Autodesk Inventor part; units mm, degrees
ref_plane "YZ Plane" through (0, 0, 0) normal (1, 0, 0) x (0, 1, 0)
ref_plane "XZ Plane" through (0, 0, 0) normal (0, 1, 0) x (-1, 0, 0)
ref_plane "XY Plane" through (0, 0, 0) normal (0, 0, 1) x (1, 0, 0)
sketch "Sketch3" plane through (0, 0, 0) normal (0, 0, 1) x (1, 0, 0)
  circle A0 centre (1.4019, 6.1779) radius 2.1844
  circle A1 centre (-11.2981, 6.1779) radius 2.1844
  circle A2 centre (-23.9981, 6.1779) radius 2.1844
  circle A3 centre (14.1019, 6.1779) radius 2.1844
  line L0 (-11.2981, 6.1779) -> (1.4019, 6.1779)
  line L1 (1.4019, 6.1779) -> (14.1019, 6.1779)
  circle A4 centre (-11.2981, 6.1779) radius 5.08
  circle A5 centre (1.4019, 6.1779) radius 5.08
  circle A6 centre (14.1019, 6.1779) radius 5.08
  line L2 (-11.2981, 11.2579) -> (1.4019, 11.2579)
  line L3 (1.4019, 11.2579) -> (14.1019, 11.2579)
  line L4 (1.4019, 6.1779) -> (1.4019, -6.5221)
  circle A7 centre (1.4019, -6.5221) radius 2.54
  circle A8 centre (1.4019, -6.5221) radius 5.08
  line L5 (-2.0302, -10.2675) -> (-18.1161, 5.8501)
  line L6 (5.1405, -9.9615) -> (17.9077, 2.813)
  point P0 (0, 0)
  point P1 (-15.8845, 3.9935)
  point P2 (18.6882, 3.9935)
  point P3 (4.8339, -10.2675)
  point P4 (-14.5389, 2.2658)
  point P5 (17.3918, 2.2658)
  point P6 (1.4019, -1.4421)
  point P7 (1.4019, 1.0979)
  point P8 (6.4819, 6.1779)
  point P9 (9.0219, 6.1779)
  point P10 (17.4689, 2.374)
  point P11 (-2.3502, -9.9468)
  point P12 (-15.2165, 2.9448)
  point P13 (-3.6781, 6.1779)
  point P14 (-6.2181, 6.1779)
  dimension "d55" = 10.16
  dimension "d54" = 10.16
  dimension "d56" = 10.16
  dimension "d59" = 4.3688
  dimension "d63" = 12.7
  dimension "d64" = 5.08
  dimension "d65" = 10.16
extrude "Extrusion7" add sketch "Sketch3" along normal blind 1.5875 contours L1 A5 L4 A0 | A0 L0 A5 L1 | A0 L4 A5 L0 | A5 L3 A6 L1 | L1 A6 L6 A8 L4 A5 | A8 | A5 L4 A8 L5 A4 L0 | L0 A4 L2 A5 | A6 L6 | A4 L5 picked at (18.1676, 5.7732) picked at (-7.2265, 5.798)
sketch "Sketch4" plane through (0, 0, 1.5875) normal (0, 0, 1) x (1, 0, 0)
  point P0 (0, 0)
properties part number "Wing poly connection"
The model under review builds one solid part; all positions refer to its coordinate system, in mm. Round coordinates to 2 decimals unless told otherwise and drop trailing zeros. Loops run counter-clockwise (first coordinate to the right, second up) from the corner with the lowest first, then second, coordinate; pieces in that order, holes last. Notation, with made-up numbers: (19, 2.25) -> (23, 2.25) arc R19 cw to (23, 32.25) -> close; hole circle Ø11 at (-1, 34.5). An arc over 180 degrees is marked (long way). One line per question, with ' | ' between items. Start each with the question number.
Item 1: Add section C-C, the plane x = 13. Write out the cut boundary in (y, z), then the cut area to 3 significant figures.
Item 2: Add section A-A, the plane y = -7. Write out the cut boundary in (x, z), then the cut area to 3 significant figures.
Item 3: For pin 1 (4 mm diameter, centred on x = 2, y = -8, fed in from -Z), flat-tipped, find the tip position at first contact; note if it passes through.
Item 4: Add section D-D, the plane z = 1.2. Write out the cut boundary in (x, y).
Item 5: Add section B-B, the plane y = 5.5. Write out the cut boundary in (x, z).
Item 6: Wall thickness on line 1 along Y through (x, z) = (2.5, 0.4); line 2 along X through (y, z) = (7.25, 1.4); line 3 along Y through (x, z) = (3, 0.75): over which ranges is each line inside the solid? List them lowest first. Write a range as [from, to].
Return value:
1) outline: (-2.1, 0) -> (4.29, 0) -> (4.29, 1.59) -> (-2.1, 1.59) -> close; (8.06, 0) -> (11.26, 0) -> (11.26, 1.59) -> (8.06, 1.59) -> close | area: 15.2 mm2
2) outline: (-5.29, 0) -> (-1.09, 0) -> (-1.09, 1.59) -> (-5.29, 1.59) -> close; (3.9, 0) -> (8.1, 0) -> (8.1, 1.59) -> (3.9, 1.59) -> close | area: 13.3 mm2
3) pin 1: stops at z = 0
4) outline: (-15.22, 2.94) -> (-2.03, -10.27) arc R5.08 ccw to (5.14, -9.96) -> (17.91, 2.81) arc R5.08 ccw to (14.1, 11.26) -> (-11.3, 11.26) arc R5.08 ccw to start; hole circle Ø4.37 at (-11.3, 6.18); hole circle Ø5.08 at (1.4, -6.52); hole circle Ø4.37 at (1.4, 6.18); hole circle Ø4.37 at (14.1, 6.18)
5) outline: (-16.33, 0) -> (-13.37, 0) -> (-13.37, 1.59) -> (-16.33, 1.59) -> close; (-9.22, 0) -> (-0.67, 0) -> (-0.67, 1.59) -> (-9.22, 1.59) -> close; (3.48, 0) -> (12.03, 0) -> (12.03, 1.59) -> (3.48, 1.59) -> close; (16.18, 0) -> (19.14, 0) -> (19.14, 1.59) -> (16.18, 1.59) -> close
6) line 1: y = [-11.48, -8.81], [-4.23, 4.29], [8.07, 11.26] | line 2: x = [-16.26, -13.2], [-9.39, -0.5], [3.31, 12.2], [16.01, 19.07] | line 3: y = [-11.34, -8.5], [-4.55, 4.69], [7.67, 11.26]
